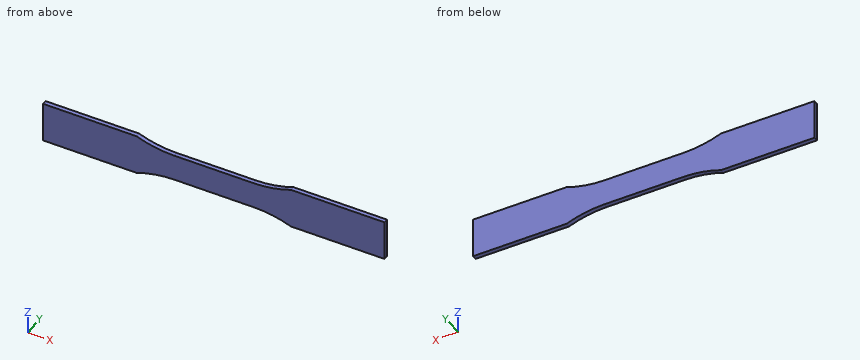
```python
from build123d import *

# Parameters (mm, degrees)
CROQUIS1_W              = 57
CROQUIS1_H              = 19
SALIENTE_EXTRUIR1_DEPTH = 1.6


with BuildPart() as part:
    # Croquis1 → Saliente-Extruir1 (new body, symmetric)
    with BuildSketch(Plane(origin=(0, 0, 0), x_dir=(1, 0, 0), z_dir=(0, 1, 0))):
        with BuildLine():
            Line((-123, -14.5), (-55.610883423, -14.5))
            ThreePointArc((-55.610883423, -14.5), (-42.284048752, -10.760452236), (-28.5, -9.5))
            Line((-28.5, -9.5), (-28.5, 9.5))
            ThreePointArc((-28.5, 9.5), (-42.284048752, 10.760452236), (-55.610883423, 14.5))
            Line((-55.610883423, 14.5), (-123, 14.5))
            Line((-123, 14.5), (-123, -14.5))
        make_face()
        with BuildLine():
            Line((55.610883423, -14.5), (123, -14.5))
            Line((123, -14.5), (123, 14.5))
            Line((123, 14.5), (55.610883423, 14.5))
            ThreePointArc((55.610883423, 14.5), (42.284048752, 10.760452236), (28.5, 9.5))
            Line((28.5, 9.5), (28.5, -9.5))
            ThreePointArc((28.5, -9.5), (42.284048752, -10.760452236), (55.610883423, -14.5))
        make_face()
        Rectangle(CROQUIS1_W, CROQUIS1_H)
    extrude(amount=SALIENTE_EXTRUIR1_DEPTH, both=True)


solid = part.part
```
Geometry check sheet. Reference: the model listing, model coordinates, mm. Round coordinates to 2 decimals unless told otherwise and drop trailing zeros. Order: outer loops, then holes, each group sorted by start corner. A loop starts at its lowest first (then second) coordinate and runs counter-clockwise, first axis right, second up. Notation, with made-up numbers: (79, 49) - (102, 49) arc R23 cw to (102, 70) - close; hole circle Ø1 at (-15.5, 11.25). An arc over 180 degrees is marked (long way). Use a Markdown table: item, result. Add a question column.
(1) Material ranges on line 1 along Z through (x, y) = (0.5, -1.3); line 2 along Z through (x, y) = (-39.5, -0.5), recorded low to high. Write a range as [from, to].
(2) Sectioned sample at B-B, the plane x = -53. Enter the section's corners in (y, z), and give its area (3 significant figures).
(3) Sectioned sample at C-C, the plane x = 42.5. Enter the section's corners in (y, z).
(4) Sectioned sample at A-A, the plane y = 0.6. Enter the section's corners in (x, z), and give its area (3 significant figures).
(5) Depth check by flat-ended pin: pin 1 (1.6 mm diameter, centred on x = -11, y = 0, fed in from +Z). Enter the tip coordinate at first touch or a pass-through.
Answers below:
| question | item | result |
|---|---|---|
| 1 | line 1 | [-9.5, 9.5] |
| 1 | line 2 | [-10.3, 10.3] |
| 2 | outline | (-1.6, -13.56) - (1.6, -13.56) - (1.6, 13.56) - (-1.6, 13.56) - close |
| 2 | area | 86.8 mm² |
| 3 | outline | (-1.6, -10.8) - (1.6, -10.8) - (1.6, 10.8) - (-1.6, 10.8) - close |
| 4 | outline | (-123, -14.5) - (-55.61, -14.5) arc R76 cw to (-28.5, -9.5) - (28.5, -9.5) arc R76 cw to (55.61, -14.5) - (123, -14.5) - (123, 14.5) - (55.61, 14.5) arc R76 cw to (28.5, 9.5) - (-28.5, 9.5) arc R76 cw to (-55.61, 14.5) - (-123, 14.5) - close |
| 4 | area | 6,200 mm² |
| 5 | pin 1 | z = 9.5 |
